The drawing under review shows one solid part. Ordinate dimensions are in mm from its lowest x, y, z. A direction names the side the tool comes from. Coordinates: 2 decimals unless noted, no trailing zeros. Loops run counter-clockwise (first coordinate to the right, second up) from the corner with the lowest first, then second, coordinate; pieces in that order, holes last. Notation, with made-up numbers: M 55,-25 L 84,-25 A22 ccw 84,9 Z; hole C 73,-14.75 d11. An arc over 180 degrees is marked long. Answer as a JSON object with one key per item and string values. Group by question number.
1. Draft analysis for pull direction Z (two halves, no side actions). For the marked faces 1, 2 and 3, state which applies: +Z half, -Z half, draft (parallel to the pull), parting line (faces both ways), or undercut.
2. Consider section A-A (z = 64). State the section outline as (x, y) points, then the cut area to 3 significant figures.
3. Machinability: for the marked faces 4, 5 and 6, which of the approach directions +Z, -Z, +X, -X, +Y, -Y give a long, thin tool a straight path to every point of the face, cutting with its end or side? Answer none if there is none.
4. Insertion check: pin 1 (2 mm diameter, centred on y = 1.5, z = 30, fed in from -X); pin 2 (5 mm diameter, centred on y = 3, z = 23, fed in from +X); pin 3 (2 mm diameter, centred on x = 37, y = 1.5, fed in from +Z). Each pin has a flat end and moves straight along its axis. Give the tip position at first contact, or say it passes through.
5. Consider section B-B (y = 8.5). State the section outline as (x, z) points.
6. To check wall thickness, follow probe 1 along X at (y, z) = (0.75, 78); probe 2 along Z at (x, y) = (69, 2.25); probe 3 along Z at (x, y) = (42, 6.75). State the ranges of each line that lie inside material, in increasing order.
7. Consider section C-C (x = 31.5). State the section outline as (y, z) points.
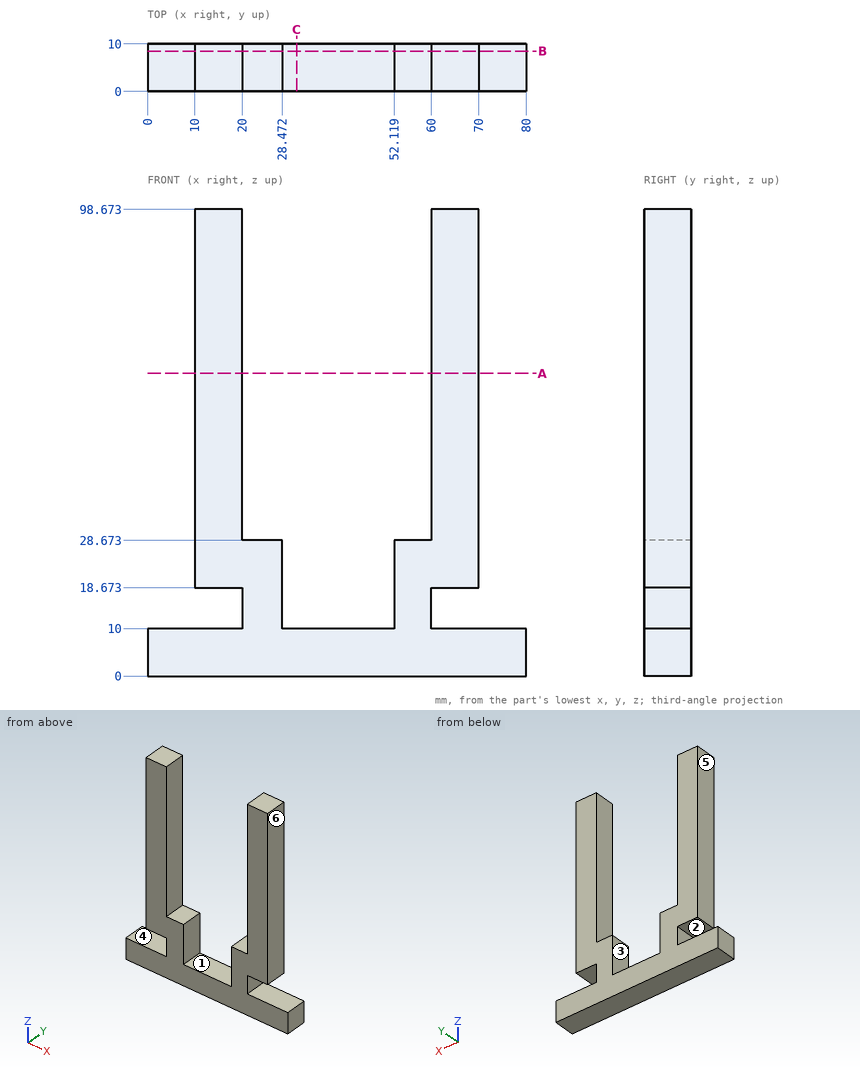
Findings below:
{
 "1": {"face 1": "+Z half", "face 2": "undercut", "face 3": "draft"},
 "2": {"outline": "M 10,0 L 20,0 L 20,10 L 10,10 Z; M 60,0 L 70,0 L 70,10 L 60,10 Z", "area": "200 mm^2"},
 "3": {"face 4": "-X, +Y, -Y", "face 5": "+Z, -X, +Y, -Y", "face 6": "+Z, +X, +Y, -Y"},
 "4": {"pin 1": "stops at x = 10", "pin 2": "stops at x = 70", "pin 3": "stops at z = 10"},
 "5": {"outline": "M 0,0 L 80,0 L 80,10 L 60,10 L 60,18.67 L 70,18.67 L 70,98.67 L 60,98.67 L 60,28.67 L 52.12,28.67 L 52.12,10 L 28.47,10 L 28.47,28.67 L 20,28.67 L 20,98.67 L 10,98.67 L 10,18.67 L 20,18.67 L 20,10 L 0,10 Z"},
 "6": {"probe 1": "x = 10 to 20, 60 to 70", "probe 2": "z = 0 to 10, 18.67 to 98.67", "probe 3": "z = 0 to 10"},
 "7": {"outline": "M 0,0 L 10,0 L 10,10 L 0,10 Z"}
}
